Model file for the job. Use its own axes, mm. A direction names the side the tool comes from. Round coordinates to 2 decimals unless told otherwise and drop trailing zeros. Loops run counter-clockwise (first coordinate to the right, second up) from the corner with the lowest first, then second, coordinate; pieces in that order, holes last. Notation, with made-up numbers: M 47,71.25 L 86,71.25 A25 ccw 86,110.25 Z; hole C 48.5,-34 d5. An arc over 180 degrees is marked long. Use a Markdown table: item, result. Add a question column.
Q1. Probe line 1 (X direction, y = -1.55, z = 2.8) (3 decimals); line 2 (Y direction, x = 2.5, z = 6); line 3 (Y direction, x = -0.25, z = 4.75). List the from-to ranges inside material, lowest first. Write a range as from..to.
Q2. Mould opens along X. For faces 4 (the face through (0, 1, -1)), 5 (the face through (0.05, 6.88, 1.55)), 6 (the face through (0.35, -0.99, 1.68)) say: +X half, -X half, draft (parallel to the pull), parting line (faces both ways), or undercut.
Q3. Cut at C-C (z = 0.75). Give the cut face in (x, y), plus the area to 3 significant figures.
Q4. Cut at A-A (x = -2.5). Give the cut face in (y, z).
Q5. Cut at B-B (y = 0.5). Give the cut face in (x, z) (3 decimals).
Q6. Pin check, flat tips, straight feed: pin 1 (1 mm diameter, centred on x = -2.5, y = 4.5, fed in from -Z); pin 2 (0.6 mm diameter, centred on x = -1.5, z = -0.5, fed in from +Y); pin 3 (1 mm diameter, centred on x = 2.5, z = 5.5, fed in from +Y); pin 4 (1.2 mm diameter, centred on x = 0.5, y = 2, fed in from +Z). Stop position of each tip, or through.
Q7. Tool access for faces 1 (the face through (0, 2, 0)), 2 (the face through (0, 0, 3)), 3 (the face through (0, 1, 6)): list every direction of +Z, -Z, +X, -X, +Y, -Y with a clear straight run to the whole face (end or side of a thin tool).
from build123d import *

# Parameters (mm, degrees)
BASE_EXTRUDE_DEPTH  = 3.36
SKETCH3_R           = 1.25
BOSS_EXTRUDE1_DEPTH = 8.14
FILLET1_R           = 1
BOSS_EXTRUDE2_START = -1
SKETCH4_R           = 4.675
BOSS_EXTRUDE2_DEPTH = 1
SKETCH5_R           = 1.675
SKETCH5_R_2         = 1.175
BOSS_EXTRUDE3_DEPTH = 2


with BuildPart() as part:
    # Sketch2 → Base-Extrude (new body)
    with BuildSketch(Plane(origin=(0, 3.36, 0), x_dir=(-1, 0, 0), z_dir=(0, 1, 0))):
        with BuildLine():
            Line((-3.743744783, 0), (3.743744783, 0))
            ThreePointArc((3.743744783, 0), (4.675, 2.8), (3.743744783, 5.6))
            Line((3.743744783, 5.6), (-3.743744783, 5.6))
            ThreePointArc((-3.743744783, 5.6), (-4.675, 2.8), (-3.743744783, 0))
        make_face()
    extrude(amount=-BASE_EXTRUDE_DEPTH)

    # Sketch3 → Boss-Extrude1 (add)
    with BuildSketch(Plane(origin=(0, 3.36, 0), x_dir=(-1, 0, 0), z_dir=(0, 1, 0))):
        with Locations(Location((0, 2.8, 0), (0, 0, 90))):
            Circle(SKETCH3_R)
    extrude(amount=BOSS_EXTRUDE1_DEPTH)

    # Fillet1
    fillet1_edges = [part.edges().sort_by_distance(p)[0] for p in [
        (0, 11.5, 1.55),
    ]]
    fillet(fillet1_edges, radius=FILLET1_R)

    # Sketch4 → Boss-Extrude2 (add)
    with BuildSketch(Plane.XZ.offset(BOSS_EXTRUDE2_START)):
        with Locations(Location((0, 2.8, 0), (0, 0, 90))):
            Circle(SKETCH4_R)
    extrude(amount=BOSS_EXTRUDE2_DEPTH)

    # Sketch5 → Boss-Extrude3 (add)
    with BuildSketch(Plane.XZ):
        with Locations(Location((0, 2.8, 0), (0, 0, 90))):
            Circle(SKETCH5_R)
        with Locations(Location((0, 2.8, 0), (0, 0, 270))):
            Circle(SKETCH5_R_2, mode=Mode.SUBTRACT)
    extrude(amount=BOSS_EXTRUDE3_DEPTH)


solid = part.part
Checked values:
| question | item | result |
|---|---|---|
| 1 | line 1 | x = -1.675..-1.175, 1.175..1.675 |
| 1 | line 2 | y = 0..1 |
| 1 | line 3 | y = 0..3.36 |
| 2 | face 4 | draft |
| 2 | face 5 | parting line |
| 2 | face 6 | undercut |
| 3 | outline | M -4.2,0 L 4.2,0 L 4.2,3.36 L -4.2,3.36 Z |
| 3 | area | 28.2 mm^2 |
| 4 | outline | M 0,-1.15 L 1,-1.15 L 1,0 L 3.36,0 L 3.36,5.6 L 1,5.6 L 1,6.75 L 0,6.75 Z |
| 5 | outline | C 0,2.8 d9.35 |
| 6 | pin 1 | passes through |
| 6 | pin 2 | stops at y = 1 |
| 6 | pin 3 | stops at y = 3.36 |
| 6 | pin 4 | stops at z = 5.6 |
| 7 | face 1 | -Z, +X, -X, +Y |
| 7 | face 2 | -Y |
| 7 | face 3 | +Z, +X, -X, +Y |
